Check sheet for the modelled part. Datum: model origin and axes. Units: mm. Face numbers are marked on the shaded views. A direction names the side the tool comes from. Give positions to 0.01 mm unless a question says otherwise; leave off trailing zeros. Order: outer loops, then holes, each group sorted by start corner. A loop starts at its lowest first (then second) coordinate and runs counter-clockwise, first axis right, second up.
from build123d import *

# Parameters (mm, degrees)
SKETCH1_W           = 1
SKETCH1_H           = 7
BOSS_EXTRUDE1_DEPTH = 5


with BuildPart() as part:
    # Sketch1 → Revolve1 (revolve)
    with BuildSketch(Plane.XY, mode=Mode.PRIVATE) as revolve1_sk:
        with Locations((0.5, 3.5)):
            Rectangle(SKETCH1_W, SKETCH1_H)
    revolve(revolve1_sk.sketch.rotate(Axis((0, 7, 0), (0, -1, 0)), 180), axis=Axis((0, 7, 0), (0, -1, 0)))

    # Sketch2 → Boss-Extrude1 (add)
    with BuildSketch(Plane.XZ):
        with BuildLine():
            Line((1, -6), (-1, -6))
            ThreePointArc((-1, -6), (-1.707106781, -5.707106781), (-2, -5))
            Line((-2, -5), (-2, 5))
            ThreePointArc((-2, 5), (-1.707106781, 5.707106781), (-1, 6))
            Line((-1, 6), (1, 6))
            ThreePointArc((1, 6), (1.707106781, 5.707106781), (2, 5))
            Line((2, 5), (2, -5))
            ThreePointArc((2, -5), (1.707106781, -5.707106781), (1, -6))
        make_face()
    extrude(amount=BOSS_EXTRUDE1_DEPTH)


solid = part.part
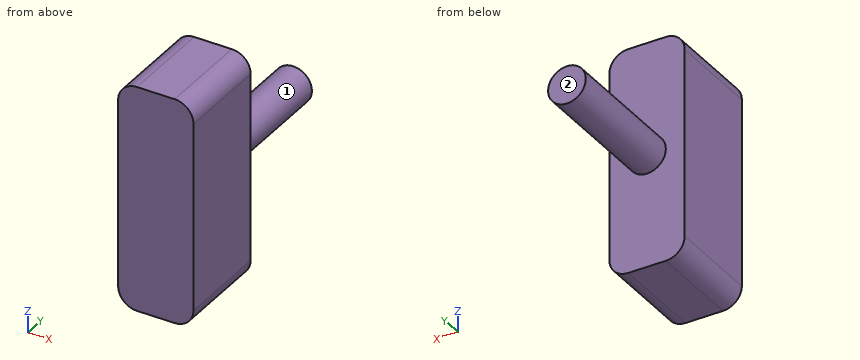
1) Section check A-A, the plane x = 0. Record the cut outline in (y, z), then the cut area to 3 significant figures.
Recorded:
outline: (-5, -6) - (0, -6) - (0, -1) - (7, -1) - (7, 1) - (0, 1) - (0, 6) - (-5, 6) - close
area: 74.0 mm2
2) Section check D-D, the plane y = 2.25. Record the cut outline in (x, z), then the cut area to 3 significant figures.
Recorded:
outline: circle Ø2 at (0, 0)
area: 3.14 mm2
3) Set-up check for the marked faces 1 and 2: record each of +Z, -Z, +X, -X, +Y, -Y from which the full face is reachable in a straight line by a thin tool's end or side.
Recorded:
face 1: +Y
face 2: +Z, -Z, +X, -X, +Y
4) Section check C-C, the plane z = 1.75. Record the cut outline in (x, y).
Recorded:
outline: (-2, -5) - (2, -5) - (2, 0) - (-2, 0) - close
5) Depth check by flat-ended pin: pin 1 Ø2 at (x, z) = (1, 2.5) entering from +Y. Enter the tip coordinate at first touch or a pass-through.
Recorded:
pin 1: stops at y = 0
6) Section check B-B, the plane y = -1.75. Record the cut outline in (x, z).
Recorded:
outline: (-2, -5) arc R1 ccw to (-1, -6) - (1, -6) arc R1 ccw to (2, -5) - (2, 5) arc R1 ccw to (1, 6) - (-1, 6) arc R1 ccw to (-2, 5) - close
7) Material ranges on L1, parallel to Y at x = -1.7, z = -4.5; L2, parallel to Z at x = -1.1, y = -1; L3, parallel to Z at x = 1.5, y = -1.75, recorded low to high.
Recorded:
L1: y = -5 to 0
L2: z = -5.99 to 5.99
L3: z = -5.87 to 5.87
